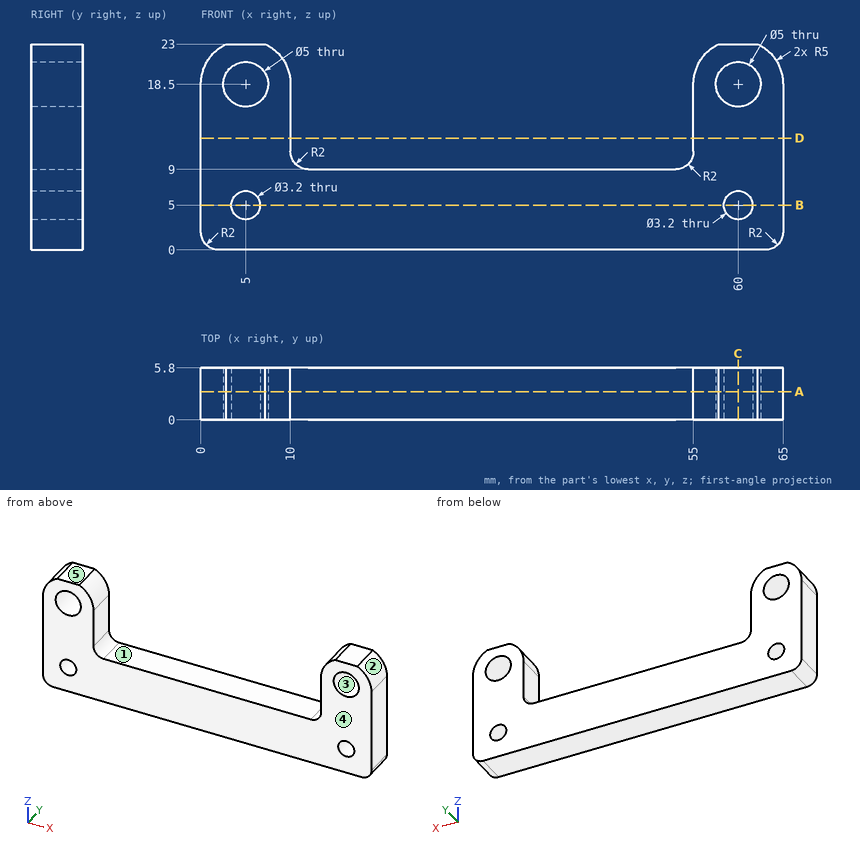
Check sheet for the drawn part. Datum: minimum x, y, z corner. Units: mm. A direction names the side the tool comes from. Round coordinates to 2 decimals unless told otherwise and drop trailing zeros. Loops run counter-clockwise (first coordinate to the right, second up) from the corner with the lowest first, then second, coordinate; pieces in that order, holes last. Notation, with made-up numbers: (18.25, 40.25) -> (43.25, 40.25) arc R27 ccw to (43.25, 59.25) -> close; hole circle Ø1 at (54.5, -24.75). An arc over 180 degrees is marked (long way). Put each result on its own line as item: value. Start each with the question number.
1. Scan lines: probe 1 along X at (y, z) = (3.2, 18.5); probe 2 along X at (y, z) = (2.8, 5); probe 3 along X at (y, z) = (2.8, 20.75). Record each from-to range of solid material in increasing order.
2. Section check D-D (z = 12.5). Enter the section's corners in (x, y).
3. Gauge pin test, flat ends, axial feed: pin 1 (3 mm diameter, centred on x = 54, y = 4.5, fed in from +Z); pin 2 (1.5 mm diameter, centred on x = 19, y = 1, fed in from +Z). Record the tip position at first contact, or that the pin passes through.
4. Section check A-A (y = 3.15). Enter the section's corners in (x, z), plus the area to 3 significant figures.
5. Access from +Z, -Z, +X, -X, +Y, -Y to the whole of each face (thin tool, end or side, straight path). Record for the marked faces 1 and 2.
6. Section check B-B (z = 5). Enter the section's corners in (x, y), plus the area to 3 significant figures.
7. Draft check along Z on the marked faces 3, 4 and 5. Enter one of: +Z half, -Z half, draft (parallel to the pull), parting line (faces both ways), or undercut.
8. Section check C-C (x = 60). Enter the section's corners in (y, z), plus the area to 3 significant figures.
Findings:
1. probe 1: x = 0 to 2.5, 7.5 to 10, 55 to 57.5, 62.5 to 65
1. probe 2: x = 0 to 3.4, 6.6 to 58.4, 61.6 to 65
1. probe 3: x = 0.53 to 3.91, 6.09 to 9.47, 55.53 to 58.91, 61.09 to 64.47
2. outline: (0, 0) -> (10, 0) -> (10, 5.8) -> (0, 5.8) -> close; (55, 0) -> (65, 0) -> (65, 5.8) -> (55, 5.8) -> close
3. pin 1: stops at z = 20.68
3. pin 2: stops at z = 9
4. outline: (0, 2) arc R2 ccw to (2, 0) -> (63, 0) arc R2 ccw to (65, 2) -> (65, 18.5) arc R5 ccw to (62.18, 23) -> (57.82, 23) arc R5 ccw to (55, 18.5) -> (55, 11) arc R2 cw to (53, 9) -> (12, 9) arc R2 cw to (10, 11) -> (10, 18.5) arc R5 ccw to (7.18, 23) -> (2.82, 23) arc R5 ccw to (0, 18.5) -> close; hole circle Ø5 at (5, 18.5); hole circle Ø3.2 at (5, 5); hole circle Ø5 at (60, 18.5); hole circle Ø3.2 at (60, 5)
4. area: 795 mm^2
5. face 1: +Z, +Y, -Y
5. face 2: +Z, +X, +Y, -Y
6. outline: (0, 0) -> (3.4, 0) -> (3.4, 5.8) -> (0, 5.8) -> close; (6.6, 0) -> (58.4, 0) -> (58.4, 5.8) -> (6.6, 5.8) -> close; (61.6, 0) -> (65, 0) -> (65, 5.8) -> (61.6, 5.8) -> close
6. area: 340 mm^2
7. face 3: undercut
7. face 4: draft
7. face 5: +Z half
8. outline: (0, 0) -> (5.8, 0) -> (5.8, 3.4) -> (0, 3.4) -> close; (0, 6.6) -> (5.8, 6.6) -> (5.8, 16) -> (0, 16) -> close; (0, 21) -> (5.8, 21) -> (5.8, 23) -> (0, 23) -> close
8. area: 85.8 mm^2
